The listing builds one solid part. Answer for the finished solid, in the listing's coordinates (mm). A direction names the side the tool comes from. Give positions to 0.01 mm unless a question says otherwise; leave off trailing zeros. Loops run counter-clockwise (first coordinate to the right, second up) from the corner with the lowest first, then second, coordinate; pieces in that order, holes last. Notation, with made-up numbers: M 84,60.5 L 89,60.5 A33 ccw 89,97.5 Z; hole C 83,52.5 d4. An arc over 180 degrees is marked long. Return JSON: item names as keys, results as strings.
from build123d import *

# Parameters (mm, degrees)
F1_DEPTH = 150
F2_W     = 100
F2_H     = 20
F3_DEPTH = 20.001
F4_W     = 20
F4_H     = 80
F6_DEPTH = 25
F7_DEPTH = 25
F8_R     = 2.5
F9_DEPTH = 20.001


with BuildPart() as f1:
    # F0 (on Front) → F1 (new body)
    with BuildSketch(Plane.XZ):
        Polygon((75, -90), (75, 90), (55, 90), (55, 10), (-25, 10), (-25, -40), (-75, -40), (-75, -90), align=None)
    extrude(amount=F1_DEPTH)

    # F2 (on face) → F3 (cut, through all)
    with BuildSketch(Plane(origin=(55, 0, 0), x_dir=(0, -1, 0), z_dir=(-1, 0, 0))):
        with Locations((78.036222, 50.444517)):
            Rectangle(F2_W, F2_H)
    extrude(amount=-F3_DEPTH, mode=Mode.SUBTRACT)

    # F4 (on face) → F6 (cut)
    with BuildSketch(Plane.XY.offset(-40)):
        with Locations((-47.512008, -75.5594)):
            Rectangle(F4_W, F4_H)
    extrude(amount=-F6_DEPTH, mode=Mode.SUBTRACT)

    # F5 (on face) → F7 (cut)
    with BuildSketch(Plane.XY.offset(-40)):
        with BuildLine():
            Line((-37.399707, -115.419537), (-37.400242, -35.966876))
            ThreePointArc((-37.400242, -35.966876), (-47.195959, -25.865494), (-57.395084, -35.5594))
            Line((-57.395084, -35.5594), (-37.512008, -35.5594))
            Line((-37.512008, -35.5594), (-37.512008, -115.5594))
            Line((-37.512008, -115.5594), (-57.398729, -115.5594))
            ThreePointArc((-57.398729, -115.5594), (-47.329774, -125.419292), (-37.399707, -115.419537))
        make_face()
    extrude(amount=-F7_DEPTH, mode=Mode.SUBTRACT)

    # F8 (on face) → F9 (cut, through all)
    with BuildSketch(Plane(origin=(55, 0, 0), x_dir=(0, -1, 0), z_dir=(-1, 0, 0))):
        with Locations((78.338511, 75.63369)):
            Circle(F8_R)
    extrude(amount=-F9_DEPTH, mode=Mode.SUBTRACT)


solid = f1.part
(1) The part is cut by section C-C (z = -47.5). Determine the outline of the cut face in (x, y), and give its area (3 significant figures).
Values follow:
{"outline": "M -75,-150 L 75,-150 L 75,0 L -75,0 Z; hole M -57.51,-115.56 L -57.4,-115.56 A10 ccw -37.4,-115.42 L -37.4,-35.97 A10 ccw -57.4,-35.56 L -57.51,-35.56 Z", "area": "20,600 mm²"}
(2) Straight lines are drawn through the part: line 1 along Z through (x, y) = (60, -43); line 2 along Z through (x, y) = (-20, -50); line 3 along Z through (x, y) = (-35.5, -96). For each, find the intervals that lie inside material, in ascending order.
Values follow:
{"line 1": "-90 to 40.44, 60.44 to 90", "line 2": "-90 to 10", "line 3": "-90 to -40"}
(3) The part is cut by section A-A (z = 57.5). Determine the outline of the cut face in (x, y).
Values follow:
{"outline": "M 55,-150 L 75,-150 L 75,-128.04 L 55,-128.04 Z; M 55,-28.04 L 75,-28.04 L 75,0 L 55,0 Z"}
(4) The part is cut by section D-D (x = -41). Determine the outline of the cut face in (y, z), and give its area (3 significant figures).
Values follow:
{"outline": "M -150,-90 L 0,-90 L 0,-40 L -28.18,-40 L -28.18,-65 L -123.1,-65 L -123.1,-40 L -150,-40 Z", "area": "5,130 mm²"}
(5) The part is cut by section B-B (y = -88). Determine the outline of the cut face in (x, z).
Values follow:
{"outline": "M -75,-90 L 75,-90 L 75,40.44 L 55,40.44 L 55,10 L -25,10 L -25,-40 L -37.4,-40 L -37.4,-65 L -57.51,-65 L -57.51,-40 L -75,-40 Z; M 55,60.44 L 75,60.44 L 75,90 L 55,90 Z"}
(6) A tool of negligible diameter and unlimited length cuts with its end or side. For faces 1 (the flat face through (65, -74, 90)), 2 (the flat face through (16, -74, 10)), 3 (the flat face through (65, -128.036, 50)), 4 (the cylindrical face through (-46.978, -25.872, -52.325)), 5 (the flat face through (-1, -74, -90)), from which of +Z, -Z, +X, -X, +Y, -Y can it reach the whole face along a straight path? Write none if from no direction.
Values follow:
{"face 1": "+Z, +X, -X, +Y, -Y", "face 2": "+Z, -X, +Y, -Y", "face 3": "+X, -X", "face 4": "+Z", "face 5": "-Z, +X, -X, +Y, -Y"}
(7) Given pin 1 (6 mm diameter, centred on x = 44.5, y = -57.5, fed in from +Z); pin 2 (6 mm diameter, centred on x = -33.5, z = -42.5, fed in from +Y); pin 3 (16 mm diameter, centred on x = -46, y = -61.5, fed in from +Z); pin 4 (3 mm diameter, centred on y = -58.5, z = 34.5, fed in from -X), each flat-ended and moving along its own axis, determine where each tip first touches the part or whether it passes through.
Values follow:
{"pin 1": "z = 10", "pin 2": "y = 0", "pin 3": "z = -65", "pin 4": "x = 55"}
(8) Determine the mould class of faces 6 (the cylindrical face through (-47.55, -125.42, -52.32)), 7 (the flat face through (55, -74, 33)), 8 (the flat face through (65, -77, 40.445)) for opening direction X: released by +X, released by -X, zero draft, split by the parting line, or undercut.
Values follow:
{"face 6": "undercut", "face 7": "released by -X", "face 8": "zero draft"}
